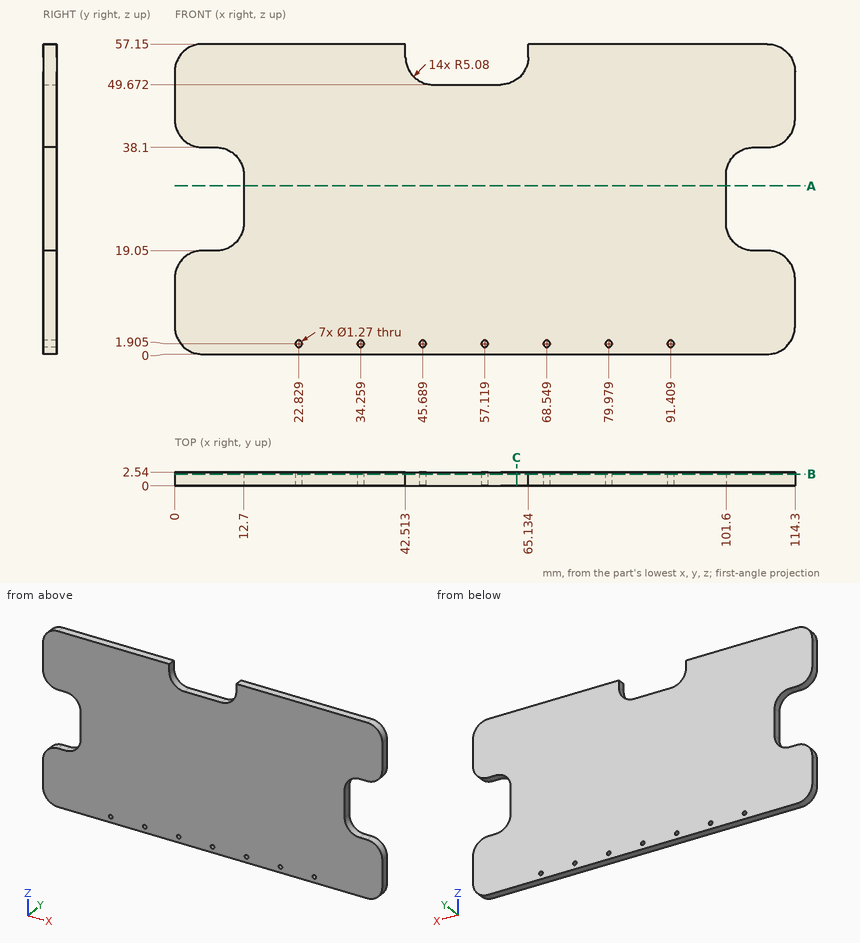
Part print with two shaded views. Sizes in mm from the minimum x, y, z corner. Give positions to 0.01 mm unless a question says otherwise; leave off trailing zeros. Loops run counter-clockwise (first coordinate to the right, second up) from the corner with the lowest first, then second, coordinate; pieces in that order, holes last. Notation, with made-up numbers: (77.25, 53) -> (120.25, 53) arc R23 cw to (120.25, 90) -> close; hole circle Ø10 at (5, 70). An arc over 180 degrees is marked (long way). One line per question, with ' | ' between items.
Q1. Cut at A-A, the plane z = 31. Write the cut outline in (x, y), plus the area to 3 significant figures.
Filled sheet:
outline: (12.7, 0) -> (101.6, 0) -> (101.6, 2.54) -> (12.7, 2.54) -> close | area: 226 mm²
Q2. Drill centre lines: line 1 along Z through (x, y) = (106.5, 0.75); line 2 along Z through (x, y) = (47.5, 2.45). Where is each one in solid material? Low to high. Write a range as [from, to].
Filled sheet:
line 1: z = [0, 19.05], [38.1, 57.15] | line 2: z = [0, 49.67]
Q3. Drop flat-ended pins along their axis: pin 1 (1.5 mm diameter, centred on y = 2, z = 39.5, fed in from -X); pin 2 (0.7 mm diameter, centred on y = 1.5, z = 55.5, fed in from -X); pin 3 (0.8 mm diameter, centred on y = 1.5, z = 28.5, fed in from -X). Give the stop position or say it passes through.
Filled sheet:
pin 1: stops at x = 0.93 | pin 2: stops at x = 1.04 | pin 3: stops at x = 12.7
Q4. Cut at B-B, the plane y = 2.15. Count the separate pieces of the cut face and the enclosed holes in it, plus the area to 3 significant figures.
Filled sheet:
separate pieces: 1 | enclosed holes: 7 | area: 5,860 mm²
Q5. Cut at C-C, the plane x = 63. Write the cut outline in (y, z).
Filled sheet:
outline: (0, 0) -> (2.54, 0) -> (2.54, 50.61) -> (0, 50.61) -> close
